Verification items for the finished model (mm, model axes). Face numbers are marked on the shaded views. A direction names the side the tool comes from. Coordinates: 2 decimals unless noted, no trailing zeros. Order: outer loops, then holes, each group sorted by start corner. A loop starts at its lowest first (then second) coordinate and runs counter-clockwise, first axis right, second up. Notation, with made-up numbers: M 47.5,81 L 61.5,81 A21 ccw 61.5,88 Z; hole C 28.5,-36 d9. An arc over 180 degrees is marked long. Return JSON: item names as keys, results as strings.
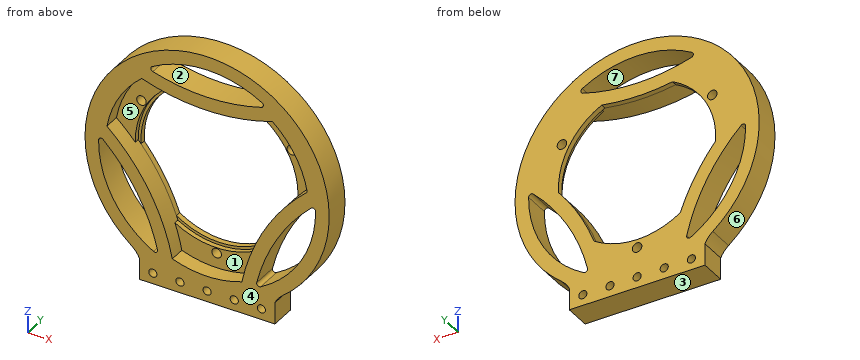
```python
from build123d import *

# Parameters (mm, degrees)
SKETCH1_R                = 37.5
BOSS_EXTRUDE1_DEPTH      = 7.6
CUT_EXTRUDE2_START       = -7.6
CUT_EXTRUDE2_DEPTH       = 7.6
SKETCH4_R                = 45
SKETCH4_R_2              = 37.5
BOSS_EXTRUDE2_DEPTH      = 7.6
SKETCH6_R                = 45
BOSS_EXTRUDE3_DEPTH      = 2
SKETCH7_R                = 1.75
CUT_EXTRUDE3_DEPTH       = 65.359614666
CIRPATTERN2_COUNT        = 3
BOSS_EXTRUDE4_START      = -9.6
BOSS_EXTRUDE4_DEPTH      = 9.6
FILLET1_R                = 10
SKETCH12_R               = 1.5
CUT_EXTRUDE6_DEPTH       = 66.773550915
LPATTERN1_COUNT          = 10
LPATTERN1_PITCH          = 10
CUT_EXTRUDE7_DEPTH       = 66.773550915
FILLET3_R                = 1
CIRPATTERN3_COUNT        = 3
FILLET3_OF_CIRPATTERN3_R = 1
BOSS_EXTRUDE5_START      = 1.8
SKETCH14_R               = 1.75
BOSS_EXTRUDE5_DEPTH      = 1.8
CIRPATTERN4_COUNT        = 3


# Read off the part's stored shape, not the designer's step: Cut-Extrude2
with BuildPart() as part:
    # Sketch1 → Boss-Extrude1 (new body)
    with BuildSketch(Plane(origin=(0, 0, 0), x_dir=(1, 0, 0), z_dir=(0, 1, 0))):
        with Locations(Location((0, 0, 0), (0, 0, 90))):
            Circle(SKETCH1_R)
    extrude(amount=BOSS_EXTRUDE1_DEPTH)

    # Cut-Extrude2 outline → Cut-Extrude2 (cut)
    with BuildSketch(Plane(origin=(0, 7.6, 0), x_dir=(1, 0, 0), z_dir=(0, 1, 0)).offset(CUT_EXTRUDE2_START)):
        with BuildLine():
            ThreePointArc((-24.104535363, -28.726666617), (0, -24.760936498), (24.104535363, -28.726666617))
            ThreePointArc((24.104535363, -28.726666617), (32.475952642, -18.75), (36.930290738, -6.511806663))
            ThreePointArc((36.930290738, -6.511806663), (21.443600029, 12.380468249), (12.825755375, 35.238473279))
            ThreePointArc((12.825755375, 35.238473279), (0, 37.5), (-12.825755375, 35.238473279))
            ThreePointArc((-12.825755375, 35.238473279), (-21.443600029, 12.380468249), (-36.930290738, -6.511806663))
            ThreePointArc((-36.930290738, -6.511806663), (-32.475952642, -18.75), (-24.104535363, -28.726666617))
        make_face()
    extrude(amount=CUT_EXTRUDE2_DEPTH, mode=Mode.SUBTRACT)

    # Sketch4 → Boss-Extrude2 (add)
    with BuildSketch(Plane(origin=(0, 0, 0), x_dir=(1, 0, 0), z_dir=(0, 1, 0))):
        with Locations(Location((0, 0, 0), (0, 0, 90))):
            Circle(SKETCH4_R)
        Circle(SKETCH4_R_2, mode=Mode.SUBTRACT)
    extrude(amount=BOSS_EXTRUDE2_DEPTH)

    # Sketch6 → Boss-Extrude3 (add)
    with BuildSketch(Plane(origin=(0, 7.6, 0), x_dir=(1, 0, 0), z_dir=(0, 1, 0))):
        with Locations(Location((0, 0, 0), (0, 0, 90))):
            Circle(SKETCH6_R)
        with BuildLine():
            ThreePointArc((-28.952849653, 1.653026611), (-25.11473671, -14.5), (-13.044861788, -25.900416617))
            ThreePointArc((-13.044861788, -25.900416617), (0, -24.760936498), (13.044861788, -25.900416617))
            ThreePointArc((13.044861788, -25.900416617), (25.11473671, -14.5), (28.952849653, 1.653026611))
            ThreePointArc((28.952849653, 1.653026611), (21.443600029, 12.380468249), (15.907987865, 24.247390006))
            ThreePointArc((15.907987865, 24.247390006), (0, 29), (-15.907987865, 24.247390006))
            ThreePointArc((-15.907987865, 24.247390006), (-21.443600029, 12.380468249), (-28.952849653, 1.653026611))
        make_face(mode=Mode.SUBTRACT)
    extrude(amount=BOSS_EXTRUDE3_DEPTH)

    # Sketch7 → Cut-Extrude3 (cut, through all)
    with BuildSketch(Plane(origin=(0, 9.6, 0), x_dir=(1, 0, 0), z_dir=(0, 1, 0))):
        with Locations(Location((0, 32, 0), (0, 0, 270))):
            Circle(SKETCH7_R)
    cut_extrude3 = extrude(amount=-CUT_EXTRUDE3_DEPTH, mode=Mode.SUBTRACT)

    # CirPattern2: Cut-Extrude3 ×3 about axis
    cirpattern2_axis = Axis((0, 0, 0), (0, 1, 0))
    for i in range(1, CIRPATTERN2_COUNT):
        add(cut_extrude3.rotate(cirpattern2_axis, i * 360 / CIRPATTERN2_COUNT), mode=Mode.SUBTRACT)

    # Sketch11 → Boss-Extrude4 (add)
    with BuildSketch(Plane(origin=(0, 9.6, 0), x_dir=(1, 0, 0), z_dir=(0, 1, 0)).offset(BOSS_EXTRUDE4_START)):
        with BuildLine():
            ThreePointArc((-22.449944321, 39), (0, 45), (22.449944321, 39))
            Line((22.449944321, 39), (25, 39))
            Line((25, 39), (25, 47))
            Line((25, 47), (-25, 47))
            Line((-25, 47), (-25, 39))
            Line((-25, 39), (-22.449944321, 39))
        make_face()
    extrude(amount=BOSS_EXTRUDE4_DEPTH)

    # Fillet1
    # the kernel refuses this fillet: 10 mm, written as the material it adds along each edge
    with BuildSketch(Plane(origin=(-22.449944321, 0, -39), x_dir=(-0.8278845523725272, 0, 0.5608985362282026), z_dir=(0, 1, 0))) as fillet1_piece_1:
        with BuildLine():
            CenterArc((7.309068463, -9.973252989), FILLET1_R, 94.191525444, 27.126753117)
            Line((2.111151705, -1.430322498), (0, 0))
            ThreePointArc((0, 0), (3.289080808, -0.12036155), (6.578161616, 0))
        make_face()
    extrude(amount=9.6)
    with BuildSketch(Plane(origin=(22.449944321, 0, -39), x_dir=(0.8278845523725283, 0, 0.560898536228201), z_dir=(0, 1, 0))) as fillet1_piece_2:
        with BuildLine():
            CenterArc((7.309068463, 9.973252989), FILLET1_R, 238.681721439, 27.126753117)
            Line((2.111151705, 1.430322498), (0, 0))
            ThreePointArc((0, 0), (3.289080808, 0.12036155), (6.578161616, 0))
        make_face()
    extrude(amount=9.6)

    # Sketch12 → Cut-Extrude6 (cut, through all)
    with BuildSketch(Plane.XZ):
        with Locations(Location((-20, -43, 0), (0, 0, 270))):
            Circle(SKETCH12_R)
    cut_extrude6 = extrude(amount=-CUT_EXTRUDE6_DEPTH, mode=Mode.SUBTRACT)

    # LPattern1: Cut-Extrude6 ×10
    with Locations(*[(i * LPATTERN1_PITCH, 0, 0) for i in range(1, LPATTERN1_COUNT)]):
        add(cut_extrude6, mode=Mode.SUBTRACT)

    # Sketch13 → Cut-Extrude7 (cut, through all)
    with BuildSketch(Plane.XZ):
        with BuildLine():
            ThreePointArc((-22.11228446, 33.332369792), (0, 29.760936498), (22.11228446, 33.332369792))
            ThreePointArc((22.11228446, 33.332369792), (0, 40), (-22.11228446, 33.332369792))
        make_face()
    cut_extrude7 = extrude(amount=-CUT_EXTRUDE7_DEPTH, mode=Mode.SUBTRACT)

    # Fillet3
    fillet3_edges = [part.edges().sort_by_distance(p)[0] for p in [
        (-22.11228446, 4.8, 33.332369792),
        (22.11228446, 4.8, 33.332369792),
    ]]
    fillet(fillet3_edges, radius=FILLET3_R)

    # CirPattern3: Cut-Extrude7 ×3 about axis
    cirpattern3_axis = Axis((0, 0, 0), (0, 1, 0))
    for i in range(1, CIRPATTERN3_COUNT):
        add(cut_extrude7.rotate(cirpattern3_axis, i * 360 / CIRPATTERN3_COUNT), mode=Mode.SUBTRACT)

    # Fillet3 of CirPattern3
    fillet3_of_cirpattern3_edges = [part.edges().sort_by_distance(p)[0] for p in [
        (39.922821238, 4.8, 2.483615182),
        (17.810536778, 4.8, -35.815984974),
        (-17.810536778, 4.8, -35.815984974),
        (-39.922821238, 4.8, 2.483615182),
    ]]
    fillet(fillet3_of_cirpattern3_edges, radius=FILLET3_OF_CIRPATTERN3_R)

    # Sketch14 → Boss-Extrude5 (add)
    with BuildSketch(Plane.XZ.offset(-7.6).offset(BOSS_EXTRUDE5_START)):
        with BuildLine():
            ThreePointArc((-15.374943027, -25.760650747), (0, -30), (15.374943027, -25.760650747))
            ThreePointArc((15.374943027, -25.760650747), (13.94564115, -30.457951205), (12.825755375, -35.238473279))
            ThreePointArc((12.825755375, -35.238473279), (0, -37.5), (-12.825755375, -35.238473279))
            ThreePointArc((-12.825755375, -35.238473279), (-13.94564115, -30.457951205), (-15.374943027, -25.760650747))
        make_face()
        with Locations(Location((0, -32, 0), (0, 0, 90))):
            Circle(SKETCH14_R, mode=Mode.SUBTRACT)
    boss_extrude5 = extrude(amount=-BOSS_EXTRUDE5_DEPTH)

    # CirPattern4: Boss-Extrude5 ×3 about axis
    cirpattern4_axis = Axis((0, 7.6, 0), (0, -1, 0))
    for i in range(1, CIRPATTERN4_COUNT):
        add(boss_extrude5.rotate(cirpattern4_axis, i * 360 / CIRPATTERN4_COUNT))


solid = part.part
```
Q1. Cross-section at C-C, the plane y = 1.75. State how many separate pieces and enclosed holes the cut face has, and give its area (3 significant figures).
Values:
{"separate pieces": "1", "enclosed holes": "9", "area": "2,470 mm^2"}
Q2. Material ranges on line 1 along X through (y, z) = (7.75, -43); line 2 along Z through (x, y) = (27, 7); line 3 along Z through (x, y) = (0.5, 2.25), recorded low to high.
Values:
{"line 1": "-25 to -21.5, -18.5 to -11.5, -8.5 to -1.5, 1.5 to 8.5, 11.5 to 18.5, 21.5 to 25", "line 2": "-36.11 to -29.51, -12.84 to -4.08, 13.08 to 14.4, 17.6 to 36", "line 3": "-47 to -44.41, -41.59 to -37.5, 24.76 to 29.76, 40 to 45"}
Q3. Draft check along X on the marked faces 4, 5, 6 and 7. Enter one of: pulls with the +X half, pulls with the -X half, needs draft (parallel to the pull), parting line crosses it, or undercut.
Values:
{"face 4": "needs draft", "face 5": "undercut", "face 6": "parting line crosses it", "face 7": "undercut"}
Q4. Cross-section at D-D, the plane z = -32. Record the boundary of the cut face in (x, y).
Values:
{"outline": "M -31.64,0 L -24,0 L -24,9.6 L -31.64,9.6 Z; M -18.71,0 L -13.55,0 L -13.55,5.8 L -1.75,5.8 L -1.75,9.6 L -18.71,9.6 Z; M 1.75,5.8 L 13.55,5.8 L 13.55,0 L 18.71,0 L 18.71,9.6 L 1.75,9.6 Z; M 24,0 L 31.64,0 L 31.64,9.6 L 24,9.6 Z"}
Q5. Cross-section at B-B, the plane z = 22.5. Record the boundary of the cut face in (x, y).
Values:
{"outline": "M -38.97,0 L -30,0 L -30,5.8 L -19.84,5.8 L -19.84,7.6 L -18.3,7.6 L -18.3,9.6 L -38.97,9.6 Z; M 18.3,7.6 L 19.84,7.6 L 19.84,5.8 L 30,5.8 L 30,0 L 38.97,0 L 38.97,9.6 L 18.3,9.6 Z"}
Q6. Go/stop test with flat-tipped pins: pin 1 (13.5 mm diameter, centred on x = -25, z = 8.5, fed in from -Y); pin 2 (2.5 mm diameter, centred on y = 3.5, z = -45, fed in from -X); pin 3 (2 mm diameter, centred on x = 17, y = 5.5, fed in from +Z). Record where each tip stops, or that it passes through.
Values:
{"pin 1": "y = 5.8", "pin 2": "x = -25", "pin 3": "z = 42.06"}
Q7. Cross-section at A-A, the plane x = 0. Record the boundary of the cut face in (y, z), and give its area (3 significant figures).
Values:
{"outline": "M 0,-47 L 9.6,-47 L 9.6,-44.5 L 0,-44.5 Z; M 0,-41.5 L 9.6,-41.5 L 9.6,-33.75 L 5.8,-33.75 L 5.8,-37.5 L 0,-37.5 Z; M 0,24.76 L 9.6,24.76 L 9.6,29.76 L 0,29.76 Z; M 0,40 L 9.6,40 L 9.6,45 L 0,45 Z; M 5.8,-30.25 L 9.6,-30.25 L 9.6,-29 L 7.6,-29 L 7.6,-30 L 5.8,-30 Z", "area": "176 mm^2"}
Q8. Tool access check on the marked faces 1, 2 and 3. Record the directions out of +Z, -Z, +X, -X, +Y, -Y that give a thin tool (end or side, any length) a straight path to the whole face; none if there is none.
Values:
{"face 1": "-Y", "face 2": "+Y, -Y", "face 3": "-Z, +X, -X, +Y, -Y"}
